Check sheet for the modelled part. Datum: model origin and axes. Units: mm. A direction names the side the tool comes from. Give positions to 0.01 mm unless a question says otherwise; leave off trailing zeros. Loops run counter-clockwise (first coordinate to the right, second up) from the corner with the lowest first, then second, coordinate; pieces in that order, holes last. Notation, with made-up numbers: (39.5, 84) - (87.5, 84) arc R16 cw to (87.5, 99) - close; hole circle Ø1 at (77, -4.75). An arc over 180 degrees is marked (long way). Answer in a Markdown table with one row per item. Add a question column.
(1) Sectioned sample at D-D on z = 22.5. Enter the section's corners in (x, y) (3 decimals).
(2) Sectioned sample at C-C on x = -0.5. Enter the section's corners in (y, z), then the cut area to 3 significant figures.
(3) Draft check along Y on faces 1 (the face through (-1, 28.5, -2)), 2 (the face through (0, -26.25, -32)), 3 (the face through (3.875, 0, 0)), 4 (the face through (0, -28.5, -1)). Enter one of: released by +Y, released by -Y, zero draft, split by the parting line, or undercut.
(4) Sectioned sample at B-B on y = 11.5. Enter the section's corners in (x, z) (3 decimals), then the cut area to 3 significant figures.
(5) Go/stop test with a flat-tipped pin: P1, Ø1.2, axis at x = -1, y = 25.5, coming from the +Z side. Record where the tip stops, or that it passes through.
(6) Sectioned sample at A-A on z = -27. Enter the section's corners in (x, y) (3 decimals), then the cut area to 3 significant figures.
(7) Set-up check for faces 5 (the face through (0, 26, 30)), 6 (the face through (0, 26.25, -32)), 7 (the face through (3, -28, 5)), 8 (the face through (-3.875, 0, 29)): record each of +Z, -Z, +X, -X, +Y, -Y from which the full face is reachable in a straight line by a thin tool's end or side.
(8) Thickness scan on L1, parallel to Y at x = 0.75, z = 8; L2, parallel to X at y = 21.5, z = -7 (3 decimals); L3, parallel to X at y = 16.5, z = -2.5 (3 decimals). Record the ranges inside material, lowest first.
from build123d import *

# Parameters (mm, degrees)
F1_DEPTH  = 3.875
F3_DEPTH  = 38
F4_W      = 27
F4_H      = 54
F4_W_2    = 20
F4_H_2    = 4
F4_W_3    = 11.7
F5_DEPTH  = 0.25
F8_R      = 0.5
F9_R      = 0.1
F11_W     = 6.75
F11_H     = 50
F12_DEPTH = 62
F14_DEPTH = 3


# Not quite as in the source:
# - a pattern or mirror of a feature is missing from the dataset's text; its kind, count and spacing are read off the source's solid


with BuildPart() as f1:
    # F0 (on Right) → F1 (new body, symmetric)
    with BuildSketch(Plane.YZ):
        Polygon((23.5, 33), (-28.5, 33), (-28.5, -33), (28.5, -33), (28.5, 30), (23.5, 30), align=None)
    extrude(amount=F1_DEPTH, both=True)

    # F2 (on face) → F3 (cut)
    with BuildSketch(Plane(origin=(0, 0, -33), x_dir=(1, 0, 0), z_dir=(0, 0, -1))):
        Polygon((3.875, 28.5), (1.875, 28.5), (3.875, 26.5), align=None)
        Polygon((3.875, -26.5), (1.875, -28.5), (3.875, -28.5), align=None)
    extrude(amount=-F3_DEPTH, mode=Mode.SUBTRACT)

    # F4 (on face) → F5 (join)
    with BuildSketch(Plane(origin=(-3.875, 0, 0), x_dir=(0, -1, 0), z_dir=(-1, 0, 0))):
        with Locations((0, 6)):
            Rectangle(F4_W, F4_H)
        with Locations((0, 29)):
            Rectangle(F4_W_2, F4_H_2, mode=Mode.SUBTRACT)
        with Locations((22.65, 6)):
            Rectangle(F4_W_3, F4_H)
        Polygon((-28.5, 30), (-28.5, -21), (-16.8, -21), (-16.8, 33), (-23.5, 33), (-23.5, 30), align=None)
    extrude(amount=F5_DEPTH)

    # F8
    f8_edges = [f1.edges().sort_by_distance(p)[0] for p in [
        (-0.125, 23.5, 33),
        (-0.125, 23.5, 30),
        (-0.125, 28.5, 30),
        (-0.125, -28.5, 33),
    ]]
    fillet(f8_edges, radius=F8_R)

    # F9
    f9_edges = [f1.edges().sort_by_distance(p)[0] for p in [
        (3.875, -2.5, 33),
        (3.875, 26, 30),
        (-4.125, 26, 30),
        (-4.125, 23.5, 31.5),
        (3.875, 23.5, 31.5),
        (-4.125, 19.9, 33),
        (-4.125, 0, 33),
        (-4.125, -22.4, 33),
        (-4.125, -28.5, 5.75),
        (3.875, -28.5, 18.75),
        (-4.125, 28.5, 4.25),
        (-4.125, -28.353553, 32.853553),
        (3.875, -28.353553, 32.853553),
        (3.875, 23.646447, 30.146447),
        (3.875, 23.353553, 32.853553),
        (3.875, 28.353553, 29.853553),
        (3.875, 28.5, 17.25),
        (-4.125, 23.353553, 32.853553),
        (-4.125, 28.353553, 29.853553),
        (-4.125, 23.646447, 30.146447),
    ]]
    fillet(f9_edges, radius=F9_R)

    # F11 (on face) → F12 (cut)
    with BuildSketch(Plane(origin=(0, 0, -33), x_dir=(1, 0, 0), z_dir=(0, 0, -1))):
        Rectangle(F11_W, F11_H)
    extrude(amount=-F12_DEPTH, mode=Mode.SUBTRACT)

    # F13 (on face) → F14 (cut)
    with BuildSketch(Plane(origin=(0, 0, -33), x_dir=(1, 0, 0), z_dir=(0, 0, -1))):
        with BuildLine():
            Line((3.375, -25), (-3.375, -25))
            Line((-3.375, -25), (-3.375, -26))
            ThreePointArc((-3.375, -26), (-3.3017766953, -26.1767766953), (-3.125, -26.25))
            Line((-3.125, -26.25), (3.125, -26.25))
            ThreePointArc((3.125, -26.25), (3.3017766953, -26.1767766953), (3.375, -26))
            Line((3.375, -26), (3.375, -25))
        make_face()
    f14 = extrude(amount=-F14_DEPTH, mode=Mode.SUBTRACT)

    # F14_copies: F14 across plane
    add(f14.mirror(Plane(origin=(0, 0, 0), x_dir=(0, 0, -1), z_dir=(0, -1, 0))), mode=Mode.SUBTRACT)


solid = f1.part
Reply:
| question | item | result |
|---|---|---|
| 1 | outline | (-4.125, -28.4) arc R0.1 ccw to (-4.025, -28.5) - (3.775, -28.5) arc R0.1 ccw to (3.875, -28.4) - (3.875, 28.4) arc R0.1 ccw to (3.775, 28.5) - (-4.025, 28.5) arc R0.1 ccw to (-4.125, 28.4) - (-4.125, 16.8) - (-3.875, 16.8) - (-3.875, 13.5) - (-4.125, 13.5) - (-4.125, -13.5) - (-3.875, -13.5) - (-3.875, -16.8) - (-4.125, -16.8) - close; hole (-3.375, -25) - (3.375, -25) - (3.375, 25) - (-3.375, 25) - close |
| 2 | outline | (-28.5, -33) - (-26.25, -33) - (-26.25, -30) - (-25, -30) - (-25, 29) - (25, 29) - (25, -30) - (26.25, -30) - (26.25, -33) - (28.5, -33) - (28.5, 29.5) arc R0.5 ccw to (28, 30) - (24, 30) arc R0.5 cw to (23.5, 30.5) - (23.5, 32.5) arc R0.5 ccw to (23, 33) - (-28, 33) arc R0.5 ccw to (-28.5, 32.5) - close |
| 2 | area | 639 mm^2 |
| 3 | face 1 | released by +Y |
| 3 | face 2 | undercut |
| 3 | face 3 | zero draft |
| 3 | face 4 | released by -Y |
| 4 | outline | (-4.125, -21) - (-3.875, -21) - (-3.875, -33) - (-3.375, -33) - (-3.375, 29) - (3.375, 29) - (3.375, -33) - (3.875, -33) - (3.875, 32.9) arc R0.1 ccw to (3.775, 33) - (-4.025, 33) arc R0.1 ccw to (-4.125, 32.9) - close |
| 4 | area | 106 mm^2 |
| 5 | P1 | z = 30 |
| 6 | outline | (-3.875, -28.5) - (1.875, -28.5) - (3.875, -26.5) - (3.875, 26.5) - (1.875, 28.5) - (-3.875, 28.5) - close; hole (-3.375, -25) - (3.375, -25) - (3.375, 25) - (-3.375, 25) - close |
| 6 | area | 100 mm^2 |
| 7 | face 5 | +Z, +X, -X, +Y |
| 7 | face 6 | -Z |
| 7 | face 7 | -Z, +X, -Y |
| 7 | face 8 | -X |
| 8 | L1 | -28.5 to -25, 25 to 28.5 |
| 8 | L2 | -4.125 to -3.375, 3.375 to 3.875 |
| 8 | L3 | -3.875 to -3.375, 3.375 to 3.875 |
